Autodesk Inventor part; units mm, degrees
ref_plane "Work Plane1" through (0, 0, 0) normal (0, 0, 1) x (1, 0, 0)
ref_plane "Work Plane2" through (0, 0, 121.25) normal (0, 0, 1) x (1, 0, 0)
ref_plane "YZ Plane" through (0, 0, 0) normal (1, 0, 0) x (0, 1, 0)
ref_plane "Work Plane1" through (0, 0, 0) normal (0, 0, 1) x (1, 0, 0)
sketch "Sketch1" plane through (0, 0, 0) normal (0, 0, 1) x (1, 0, 0)
  line L0 (10, 0) -> (-1.5, 0)
  line L1 (10, 45.2667) -> (10, 0)
  arc A0 (13.0769, 49.8821) -> (10, 45.2667) centre (15, 45.2667) ccw
  line L2 (54.8615, 67.2923) -> (13.0769, 49.8821)
  line L3 (50.4385, 77.9077) -> (54.8615, 67.2923)
  line L4 (50.4385, 77.9077) -> (29.2692, 69.0872)
  arc A1 (29.2692, 69.0872) -> (-1.5, 22.9333) centre (48.5, 22.9333) ccw
  line L5 (-1.5, 0) -> (-1.5, 22.9333)
  line L6 (15, 45.2667) -> (6.8975, 50.6683)
  line L7 (10, 48.6) -> (19.7692, 25.1538)
  line L8 (35.4, 31.6667) -> (10, 21.0833)
  line L9 (19.1124, 26.7302) -> (10, 22.9333)
  line L10 (-1.5, 22.9333) -> (10, 22.9333)
  line L11 (-1.5, 22.9333) -> (0, 22.9333)
  line L12 (0, 22.9333) -> (0, -23.4445)
  line L13 (0, -23.4445) -> (-1.5, -23.4445)
  line L14 (-1.5, -23.4445) -> (-1.5, 22.9333)
  line L15 (0, 0.0333) -> (4, 0.0333)
  line L16 (4, 0.0333) -> (10, 6.0333)
  point P0 (0, 0)
  point P1 (10.4897, 47.4247)
  point P2 (10.8397, 48.0402)
  point P3 (10, 48.6)
  point P4 (0, 22.9333)
  dimension "d3" = 1.5
  dimension "d4" = 4
  dimension "d5" = 45
  dimension "d6" = 22.9
extrude "Extrusion1" add sketch "Sketch1" along normal blind 242.5 contours L16 L15 L12 L10 L1 | A1 L6 L7 A0 L1 L10 | L1 A0 L7 L9 | L6 A0 L7
sketch "Sketch2" plane through (6.8975, 50.6683, 242.5) normal (0.5547002, 0.8320503, 0) x (0.8320503, -0.5547002, 0)
  line L0 (4.738, 242.5) -> (0, 242.5)
  line L1 (0, 242.5) -> (0, 0)
  line L2 (4.738, 0) -> (0, 0)
  line L3 (4.738, 242.5) -> (4.738, 0)
  circle A0 centre (2.5, 227.5) radius 1.25
  circle A1 centre (2.5, 177.5) radius 1.25
  circle A2 centre (2.5, 127.5) radius 1.25
  circle A3 centre (2.5, 77.5) radius 1.25
  circle A4 centre (2.5, 27.5) radius 1.25
  point P0 (22.3667, 242.5)
  dimension "d7" = 2.5
  dimension "d8" = 2.5
  dimension "d9" = 15
  dimension "d12" = 50
extrude "Extrusion2" cut sketch "Sketch2" against normal blind 3 contours A0 | A1 | A2 | A3 | A4
sketch "Sketch3" plane through (0, 0, 0) normal (0, 0, -1) x (-1, 0, 0)
  line L0 (-10, 6.0333) -> (-10, 22.9333)
  line L1 (-4, 0.0333) -> (-10, 6.0333)
  line L2 (0, 0.0333) -> (-4, 0.0333)
  line L3 (0, 22.9333) -> (0, 0.0333)
  line L4 (1.5, 22.9333) -> (0, 22.9333)
  arc A0 (1.5, 22.9333) -> (-6.8975, 50.6683) centre (-48.5, 22.9333) ccw
  line L5 (-10.8397, 48.0402) -> (-6.8975, 50.6683)
  arc A1 (-10.4897, 47.4247) -> (-10.8397, 48.0402) centre (-15, 45.2667) ccw
  line L6 (-19.1124, 26.7302) -> (-10.4897, 47.4247)
  line L7 (-10, 22.9333) -> (-19.1124, 26.7302)
  line L8 (-12.4384, 34.9479) -> (-14.7461, 29.4095)
  line L9 (-14.7461, 29.4095) -> (-11.9768, 28.2556)
  line L10 (-11.9768, 28.2556) -> (-9.6691, 33.7941)
  line L11 (-9.6691, 33.7941) -> (-12.4384, 34.9479)
  point P0 (0, 0)
  dimension "d19" = 12.7
  dimension "d20" = 6
  dimension "d21" = 3
  dimension "d22" = 3
extrude "Extrusion3" cut sketch "Sketch3" against normal blind 30 contours L11 L10 L9 L8
sketch "Sketch4" plane through (10.4897, 47.4247, 242.5) normal (0.9230769, 0.3846154, 0) x (0, 0, -1)
  line L0 (242.5, -22.4191) -> (242.5, 0)
  line L1 (242.5, 0) -> (0, 0)
  line L2 (0, -22.4191) -> (0, 0)
  line L3 (242.5, -22.4191) -> (0, -22.4191)
  line L4 (242.5, -18.2665) -> (242.5, -12.2665) construction
  line L5 (242.5, -18.2665) -> (212.5, -18.2665)
  line L6 (212.5, -18.2665) -> (212.5, -12.2665)
  line L7 (242.5, -12.2665) -> (212.5, -12.2665)
  circle A0 centre (216.1, -15.2665) radius 1.65
  line L8 (217.7743, -18.1665) -> (214.4257, -18.1665)
  line L9 (214.4257, -18.1665) -> (212.7514, -15.2665)
  line L10 (212.7514, -15.2665) -> (214.4257, -12.3665)
  line L11 (214.4257, -12.3665) -> (217.7743, -12.3665)
  line L12 (217.7743, -12.3665) -> (219.4486, -15.2665)
  line L13 (219.4486, -15.2665) -> (217.7743, -18.1665)
  point P0 (242.5, -39.7422)
  point P1 (212.5, -15.2665)
  dimension "d25" = 3.3
  dimension "d26" = 3.6
  dimension "d27" = 5.8
extrude "Extrusion4" cut sketch "Sketch4" against normal through all contours A0
ref_plane "Work Plane2" through (0, 0, 121.25) normal (0, 0, 1) x (1, 0, 0)
mirror "Mirror1" about plane through (0, 0, 121.25) normal (0, 0, 1) of "Extrusion4", "Extrusion3"
chamfer "Chamfer1" distance 3 angle 45 1 edges at (19.1124, 26.7302, 121.25)
chamfer "Chamfer2" distance 3 angle 45 2 edges at (17.1509, 27.5379, 0) (17.1509, 27.5379, 242.5)
properties part number "ESQUINA_REDONDEADA_R50_P2"
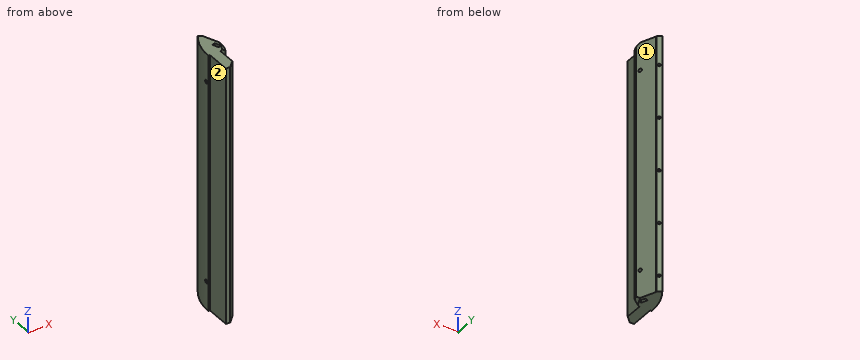
Design review of the part built by this model. Coordinates are the model's own, in mm. Face numbers are marked on the shaded views. Round coordinates to 2 decimals unless told otherwise and drop trailing zeros. Order: outer loops, then holes, each group sorted by start corner. A loop starts at its lowest first (then second) coordinate and runs counter-clockwise, first axis right, second up. Notation, with made-up numbers: (40, 30.5) - (46, 30.5) arc R18 ccw to (46, 44.5) - close; hole circle Ø2 at (84, -34). An arc over 180 degrees is marked (long way). One line per question, with ' | ' between items.
Item 1: Take a section at C-C, the plane y = 39.5. Write out the cut boundary in (x, z), then the cut area to 3 significant figures.
Checks:
outline: (1.32, 0) - (13.79, 0) - (13.79, 242.5) - (1.32, 242.5) - close | area: 3,020 mm²
Item 2: Wall thickness on line 1 (X direction, y = 11, z = 38); line 2 (Y direction, x = 6.25, z = 21); line 3 (Y direction, x = 2.25, z = 208.5): over which ranges is each line inside the solid? List them lowest first. Write a range as [from, to].
Checks:
line 1: [0, 10] | line 2: [2.28, 49.67] | line 3: [0.03, 41.93]
Item 3: For P1, Ø2.5, axis at x = 12.5, y = 30.5, coming from the +Z side; P2, Ø25, axis at y = 7, z = 165.5, coming from the -X side; P3, Ø8, axis at x = 6, z = 152.5, coming from the +Y side, all flat-tipped, find the tip position at first contact; note any pin that passes through.
Checks:
P1: z = 212.5 | P2: x = 0 | P3: y = 50.67
Item 4: Take a section at A-A, the plane z = 48. Write out the cut boundary in (x, y).
Checks:
outline: (-1.5, 22.93) - (0, 22.93) - (0, 0.03) - (4, 0.03) - (10, 6.03) - (10, 22.93) - (16.34, 25.58) - (17.96, 29.5) - (10.49, 47.42) arc R5 cw to (10.84, 48.04) - (6.9, 50.67) arc R50 ccw to start
Item 5: Draft analysis for pull direction X (two halves, no side actions). For the marked faces 1 and 2, state which applies: +X half, -X half, draft (parallel to the pull), parting line (faces both ways), or undercut.
Checks:
face 1: +X half | face 2: -X half
Item 6: Take a section at B-B, the plane y = 13.5. Write out the cut boundary in (x, z).
Checks:
outline: (0, 0) - (10, 0) - (10, 242.5) - (0, 242.5) - close
